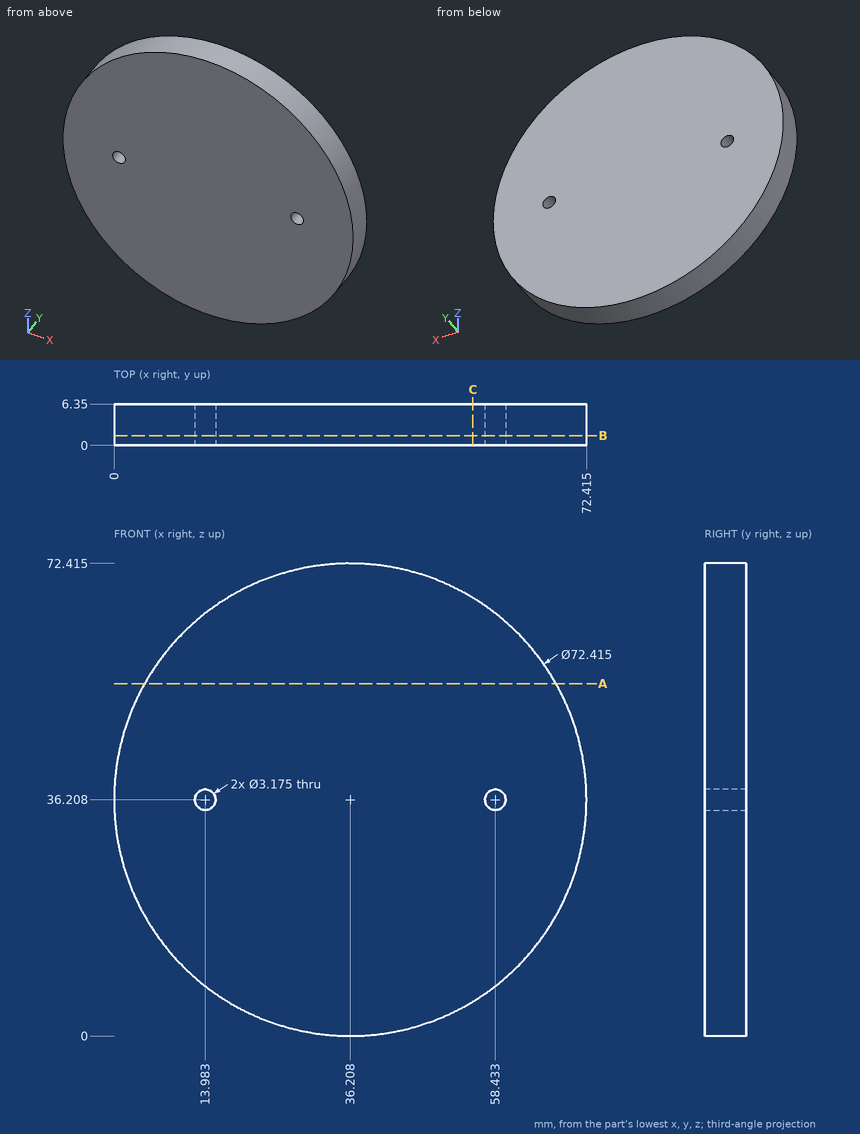
Could you check a few things on this drawing? It's one solid part, dimensions in mm from its lowest x, y, z. Give positions to 0.01 mm unless a question says otherwise; leave off trailing zeros. Order: outer loops, then holes, each group sorted by start corner. A loop starts at its lowest first (then second) coordinate and runs counter-clockwise, first axis right, second up. Notation, with made-up numbers: (62.25, -25.75) -> (86.25, -25.75) arc R24 cw to (86.25, 4.25) -> close; hole circle Ø8 at (15.25, -9.75). An arc over 180 degrees is marked (long way). Use CSV: the item, a comma, the result in double quotes. Start each with the question number.
Item 1: I'm going to push flat-ended pins straight in: P1, Ø1.9, axis at x = 58.43, z = 36.21, coming from the +Y side; P2, Ø3.5, axis at x = 13.98, z = 36.21, coming from the +Y side; P3, Ø2, axis at x = 52, y = 5, coming from the -Z side. Where does each tip first touch, or does it pass through?
Item 2: If I drill on probe 1 along Z at (x, y) = (59.5, 4) (1 decimal); probe 2 along Z at (x, y) = (57.5, 0.5) (1 decimal); probe 3 along Z at (x, y) = (44, 6), over which ranges is the centre line in solid material (lowest first)? Write a range as [from, to].
Item 3: Suppose I cut it at C-C (x = 55). List the corners of the cut face in (y, z) for me.
Item 4: Suppose I cut it at A-A (z = 54). List the corners of the cut face in (x, y) for me.
Item 5: Suppose I cut it at B-B (y = 1.5). List the corners of the cut face in (x, z) for me (1 decimal), and give its area (3 significant figures).
Answer block:
1,P1,"passes through"
1,P2,"stops at y = 6.35"
1,P3,"stops at z = 3.16"
2,probe 1,"z = [8.5, 35], [37.4, 63.9]"
2,probe 2,"z = [6.9, 34.9], [37.5, 65.5]"
2,probe 3,"z = [0.85, 71.57]"
3,outline,"(0, 5.26) -> (6.35, 5.26) -> (6.35, 67.16) -> (0, 67.16) -> close"
4,outline,"(4.67, 0) -> (67.74, 0) -> (67.74, 6.35) -> (4.67, 6.35) -> close"
5,outline,"circle Ø72.4 at (36.2, 36.2); hole circle Ø3.2 at (14, 36.2); hole circle Ø3.2 at (58.4, 36.2)"
5,area,"4,100 mm^2"
